```python
from build123d import *

# Parameters (mm, degrees)
BOSS_EXTRUDE1_DEPTH     = 127
SKETCH2_R               = 3.175
CUT_EXTRUDE1_DEPTH      = 25.4
SKETCH3_R               = 3.175
CUT_EXTRUDE2_DEPTH      = 1
CUT_EXTRUDE2_DEPTH_BACK = 26.4


with BuildPart() as part:
    # Sketch1 → Boss-Extrude1 (new body)
    with BuildSketch(Plane(origin=(0, 0, 0), x_dir=(1, 0, 0), z_dir=(0, 1, 0))):
        with BuildLine():
            Line((4, 0), (21.4, 0))
            ThreePointArc((21.4, 0), (24.228427125, 1.171572875), (25.4, 4))
            Line((25.4, 4), (25.4, 21.4))
            ThreePointArc((25.4, 21.4), (24.228427125, 24.228427125), (21.4, 25.4))
            Line((21.4, 25.4), (4, 25.4))
            ThreePointArc((4, 25.4), (1.171572875, 24.228427125), (0, 21.4))
            Line((0, 21.4), (0, 4))
            ThreePointArc((0, 4), (1.171572875, 1.171572875), (4, 0))
        make_face()
        with BuildLine():
            Line((20.86, 2.54), (4.54, 2.54))
            ThreePointArc((4.54, 2.54), (3.125786438, 3.125786438), (2.54, 4.54))
            Line((2.54, 4.54), (2.54, 20.86))
            ThreePointArc((2.54, 20.86), (3.125786438, 22.274213562), (4.54, 22.86))
            Line((4.54, 22.86), (20.86, 22.86))
            ThreePointArc((20.86, 22.86), (22.274213562, 22.274213562), (22.86, 20.86))
            Line((22.86, 20.86), (22.86, 4.54))
            ThreePointArc((22.86, 4.54), (22.274213562, 3.125786438), (20.86, 2.54))
        make_face(mode=Mode.SUBTRACT)
    extrude(amount=BOSS_EXTRUDE1_DEPTH)

    # Sketch2 → Cut-Extrude1 (cut)
    with BuildSketch(Plane(origin=(0, 0, 0), x_dir=(0, 0, -1), z_dir=(1, 0, 0))):
        with Locations((12.9921, 7.9375)):
            Circle(SKETCH2_R)
        with Locations((12.9921, 119.0625)):
            Circle(SKETCH2_R)
    extrude(amount=CUT_EXTRUDE1_DEPTH, mode=Mode.SUBTRACT)

    # Sketch3 → Cut-Extrude2 (cut, two sides)
    with BuildSketch(Plane(origin=(0, 0, -25.4), x_dir=(-1, 0, 0), z_dir=(0, 0, -1))) as cut_extrude2_sk:
        with Locations((-12.699512574, 88.9)):
            Circle(SKETCH3_R)
        with Locations((-12.699512574, 63.5)):
            Circle(SKETCH3_R)
        with Locations((-12.699512574, 38.1)):
            Circle(SKETCH3_R)
    extrude(amount=CUT_EXTRUDE2_DEPTH, mode=Mode.SUBTRACT)
    extrude(cut_extrude2_sk.sketch, amount=-CUT_EXTRUDE2_DEPTH_BACK, mode=Mode.SUBTRACT)


solid = part.part
```
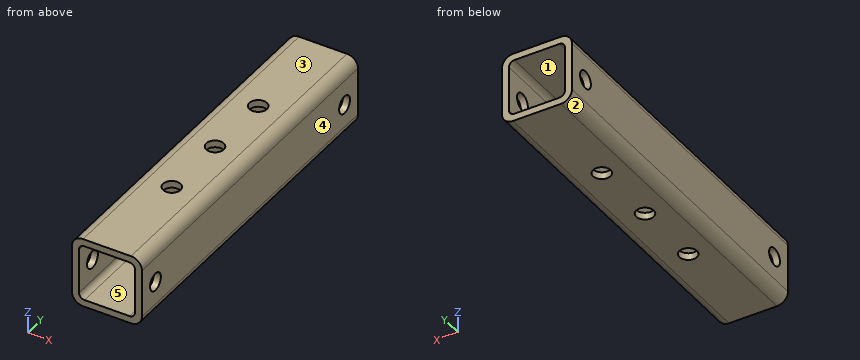
Here's how the part is built. I have some questions about the finished solid (model axes, mm). Face numbers are marked on the shaded views. A direction names the side the tool comes from. Round coordinates to 2 decimals unless told otherwise and drop trailing zeros. Loops run counter-clockwise (first coordinate to the right, second up) from the corner with the lowest first, then second, coordinate; pieces in that order, holes last.
1. Suppose I cut it at A-A, the plane z = -17.25. Please give me the cut outline in (x, y), and give its area (3 significant figures).
Answers:
outline: (0, 0) - (2.54, 0) - (2.54, 127) - (0, 127) - close; (22.86, 0) - (25.4, 0) - (25.4, 127) - (22.86, 127) - close
area: 645 mm2
2. Suppose I cut it at D-D, the plane x = 12.75. Give the number of separate pieces and of enclosed holes in the cut face, and give its area (3 significant figures).
Answers:
separate pieces: 8
enclosed holes: 0
area: 548 mm2
3. Thinking about a two-plate mould opening in Z: for the marked faces 1, 2 and 3, which applies, released by +Z, released by -Z, zero draft, split by the parting line, or undercut?
Answers:
face 1: undercut
face 2: released by -Z
face 3: released by +Z
4. Suppose I cut it at C-C, the plane x = 19.25. Please give me the cut outline in (y, z).
Answers:
outline: (0, -25.4) - (127, -25.4) - (127, -22.86) - (0, -22.86) - close; (0, -2.54) - (127, -2.54) - (127, 0) - (0, 0) - close
5. If I drill on probe 1 along Z at (x, y) = (14.5, 10.5); probe 2 along X at (y, z) = (24.5, -6.75); probe 3 along Z at (x, y) = (21.25, 105), over which ranges is the centre line in solid material (lowest first)?
Answers:
probe 1: z = -25.4 to -22.86, -2.54 to 0
probe 2: x = 0 to 2.54, 22.86 to 25.4
probe 3: z = -25.4 to -22.82, -2.58 to 0
6. For the marked faces 4 and 5, which set-ups out of +Z, -Z, +X, -X, +Y, -Y let a thin tool reach every point of the face, with its end or its side?
Answers:
face 4: +Z, -Z, +X, +Y, -Y
face 5: +Y, -Y
7. Suppose I cut it at B-B, the plane y = 73. Please give me the cut outline in (x, z), and give its area (3 significant figures).
Answers:
outline: (0, -21.4) arc R4 ccw to (4, -25.4) - (21.4, -25.4) arc R4 ccw to (25.4, -21.4) - (25.4, -4) arc R4 ccw to (21.4, 0) - (4, 0) arc R4 ccw to (0, -4) - close; hole (2.54, -20.86) arc R2 ccw to (4.54, -22.86) - (20.86, -22.86) arc R2 ccw to (22.86, -20.86) - (22.86, -4.54) arc R2 ccw to (20.86, -2.54) - (4.54, -2.54) arc R2 ccw to (2.54, -4.54) - close
area: 222 mm2
8. Will these pins go through, and if not, where does the flat tip stop? pin 1 (5 mm diameter, centred on y = 7.94, z = -12.99, fed in from +X); pin 2 (1.5 mm diameter, centred on x = 3, y = 35, fed in from -Z).
Answers:
pin 1: passes through
pin 2: stops at z = -25.39
